```python
from build123d import *

# Parameters (mm, degrees)
F0_R     = 33.02
F1_DEPTH = 10.16
F2_R     = 5.08
F3_W     = 5.08
F3_H     = 5.08
F4_DEPTH = 7.62
F5_W     = 18.572674
F5_H     = 5.08
F6_DEPTH = 2.54
F7_W     = 73.66
F7_H     = 10.16
F8_DEPTH = 2.032


with BuildPart() as f1:
    # F0 (on Top) → F1 (new body)
    with BuildSketch(Plane.XY):
        Circle(F0_R)
    extrude(amount=F1_DEPTH)

    # F2
    f2_edges = [f1.edges().sort_by_distance(p)[0] for p in [
        (-33.02, 0, 10.16),
    ]]
    fillet(f2_edges, radius=F2_R)

    # F3 (on face) → F4 (join)
    with BuildSketch(Plane.XY.offset(10.16)):
        Rectangle(F3_W, F3_H)
    extrude(amount=F4_DEPTH)

    # F5 (on face) → F6 (join)
    with BuildSketch(Plane.XY.offset(17.78)):
        Rectangle(F5_W, F5_H)
    extrude(amount=F6_DEPTH)

    # F7 (on Top) → F8 (join)
    with BuildSketch(Plane.XY):
        Rectangle(F7_W, F7_H)
    extrude(amount=F8_DEPTH)


solid = f1.part
```
Check sheet for the modelled part. Datum: model origin and axes. Units: mm. A direction names the side the tool comes from. Coordinates: 2 decimals unless noted, no trailing zeros. Order: outer loops, then holes, each group sorted by start corner. A loop starts at its lowest first (then second) coordinate and runs counter-clockwise, first axis right, second up. Notation, with made-up numbers: (23.5, -7.5) -> (80.5, -7.5) arc R21 cw to (80.5, 2.5) -> close; hole circle Ø10 at (80, 31). An arc over 180 degrees is marked (long way). Write item = value, one per line. Start each with the question number.
1) Cross-section at A-A (y = 0). Enter the section's corners in (x, z), then the cut area to 3 significant figures.
2) Material ranges on L1, parallel to Z at x = -21, y = -3.5; L2, parallel to Y at x = 0.5, z = 4; L3, parallel to Z at x = -34, y = 5, recorded low to high.
3) Access from +Z, -Z, +X, -X, +Y, -Y to the whole of each face (thin tool, end or side, straight path). Record for faces 4 (the flat face through (2.54, 0, 14)), 5 (the flat face through (-35, 5.08, 1)), 6 (the flat face through (-35, -5.08, 1)).
4) Mould release check, pull along Z, two halves, no side actions. Record for faces 1 (the flat face through (35, 0, 2.032)), 2 (the flat face through (0, 2.54, 16)), 3 (the flat face through (-6, 0, 17.78)): +Z half, -Z half, draft (parallel to the pull), parting line (faces both ways), or undercut.
5) Cross-section at B-B (x = 0). Enter the section's corners in (y, z).
6) Cross-section at C-C (z = 12). Enter the section's corners in (x, y).
7) Go/stop test with flat-tipped pins: P1, Ø3, axis at y = -0.5, z = 18.5, coming from the +X side; P2, Ø1.5, axis at y = 0.5, z = 15, coming from the -X side; P3, Ø4, axis at x = 24.5, y = 23, coming from the +Z side; P4, Ø1.5, axis at x = 5.5, y = 0, coming from the -Z side. Record where each tip stops, or that it passes through.
Ans:
q1.outline = (-36.83, 0) -> (36.83, 0) -> (36.83, 2.03) -> (33.02, 2.03) -> (33.02, 5.08) arc R5.08 ccw to (27.94, 10.16) -> (2.54, 10.16) -> (2.54, 17.78) -> (9.29, 17.78) -> (9.29, 20.32) -> (-9.29, 20.32) -> (-9.29, 17.78) -> (-2.54, 17.78) -> (-2.54, 10.16) -> (-27.94, 10.16) arc R5.08 ccw to (-33.02, 5.08) -> (-33.02, 2.03) -> (-36.83, 2.03) -> close
q1.area = 761 mm²
q2.L1 = 0 to 10.16
q2.L2 = -33.02 to 33.02
q2.L3 = 0 to 2.03
q3.face_4 = +X, +Y, -Y
q3.face_5 = +Z, -Z, -X, +Y
q3.face_6 = +Z, -Z, -X, -Y
q4.face_1 = +Z half
q4.face_2 = draft
q4.face_3 = undercut
q5.outline = (-33.02, 0) -> (33.02, 0) -> (33.02, 5.08) arc R5.08 ccw to (27.94, 10.16) -> (2.54, 10.16) -> (2.54, 20.32) -> (-2.54, 20.32) -> (-2.54, 10.16) -> (-27.94, 10.16) arc R5.08 ccw to (-33.02, 5.08) -> close
q6.outline = (-2.54, -2.54) -> (2.54, -2.54) -> (2.54, 2.54) -> (-2.54, 2.54) -> close
q7.P1 = 9.29
q7.P2 = -2.54
q7.P3 = 8.6
q7.P4 = 0
